Part model, mm, in its own coordinate system. Coordinates: 2 decimals unless noted, no trailing zeros. Loops run counter-clockwise (first coordinate to the right, second up) from the corner with the lowest first, then second, coordinate; pieces in that order, holes last. Notation, with made-up numbers: (44, 1) - (96, 1) arc R18 ccw to (96, 10) - close; hole circle Ø5 at (47, 57). An arc over 180 degrees is marked (long way). Use a Markdown table: item, result. Add a question column.
1) Band-saw the part on A-A (x = 64). Give the cut face in (y, z), plus the area to 3 significant figures.
2) Band-saw the part on D-D (y = 8). Give the cut face in (x, z).
3) Probe probe 1 along X at (y, z) = (1.5, 2); probe 2 along X at (y, z) = (-4.5, 9.5); probe 3 along Y at (x, z) = (31.5, 5). List the from-to ranges inside material, lowest first. Write a range as [from, to].
4) Pull direction Y, two halves, no side cores. Call faces 1 (the face through (30.03, 0.51, 0.23)), 2 (the face through (-34.713, -0.375, 0.231)), 3 (the face through (21, 0, 16.5)): +Y half, -Y half, draft (parallel to the pull), parting line (faces both ways), or undercut.
5) Drop flat-ended pins along their axis: P1, Ø4, axis at x = 63.04, y = 3.51, coming from the +Z side; P2, Ø1.5, axis at x = -16.5, z = -10, coming from the -Y side; P3, Ø10, axis at x = -15.5, z = 2, coming from the +Y side; P4, Ø1.5, axis at x = 14.5, z = 12.5, coming from the -Y side. Give the stop position or say it passes through.
6) Band-saw the part on C-C (x = 7.5). Give the cut face in (y, z).
7) Band-saw the part on B-B (z = 8). Give the cut face in (x, y) (3 decimals).
from build123d import *

# Parameters (mm, degrees)
SALIENTE_EXTRUIR1_DEPTH = 16.5
CROQUIS2_R              = 3.175
CORTAR_EXTRUIR1_DEPTH   = 90.961328235


with BuildPart() as part:
    # Croquis1 → Saliente-Extruir1 (new, symmetric)
    with BuildSketch(Plane.XY):
        Polygon((-37.85864365, 29.585656648), (73.418614151, 23.179824137), (78.286202478, -23.179824137), (-31.65396053, -29.508684898), align=None)
    extrude(amount=SALIENTE_EXTRUIR1_DEPTH, both=True)

    # Croquis2 → Cortar-Extruir1 (cut, through all)
    with BuildSketch(Plane.XY.offset(16.5)):
        with Locations((63.036149834, 3.50684658)):
            Circle(CROQUIS2_R)
        with Locations((33.200158154, 0.374179913)):
            Circle(CROQUIS2_R)
        with Locations((8.09814382, -2.261436976)):
            Circle(CROQUIS2_R)
        with Locations((-21.73784786, -5.394103642)):
            Circle(CROQUIS2_R)
    extrude(amount=-CORTAR_EXTRUIR1_DEPTH, mode=Mode.SUBTRACT)


solid = part.part
Answer block:
| question | item | result |
|---|---|---|
| 1 | outline | (-24, -16.5) - (0.48, -16.5) - (0.48, 16.5) - (-24, 16.5) - close; (6.53, -16.5) - (23.72, -16.5) - (23.72, 16.5) - (6.53, 16.5) - close |
| 1 | area | 1,380 mm2 |
| 2 | outline | (-35.59, -16.5) - (75.01, -16.5) - (75.01, 16.5) - (-35.59, 16.5) - close |
| 3 | probe 1 | [-34.91, 30.23], [36.17, 60.58], [65.5, 75.69] |
| 3 | probe 2 | [-34.28, -24.78], [-18.69, 5.85], [10.35, 76.32] |
| 3 | probe 3 | [-25.87, -2.31], [3.06, 25.59] |
| 4 | face 1 | undercut |
| 4 | face 2 | -Y half |
| 4 | face 3 | draft |
| 5 | P1 | through |
| 5 | P2 | y = -28.68 |
| 5 | P3 | y = 28.59 |
| 5 | P4 | y = -26.89 |
| 6 | outline | (-27.25, -16.5) - (-5.38, -16.5) - (-5.38, 16.5) - (-27.25, 16.5) - close; (0.86, -16.5) - (26.97, -16.5) - (26.97, 16.5) - (0.86, 16.5) - close |
| 7 | outline | (-37.859, 29.586) - (-31.654, -29.509) - (78.286, -23.18) - (73.419, 23.18) - close; hole circle Ø6.35 at (-21.738, -5.394); hole circle Ø6.35 at (8.098, -2.261); hole circle Ø6.35 at (33.2, 0.374); hole circle Ø6.35 at (63.036, 3.507) |
